from build123d import *

# Parameters (mm, degrees)
F0_R        = 5.8
F0_R_2      = 1.1
F1_DEPTH    = 2.5
F2_R        = 0.65
F3_DEPTH    = 25
F5_T2_ANGLE = 77.9776147156
F5_T4_ANGLE = 162.2494051266
F5_T6_ANGLE = 155.9758879551
F5_T8_ANGLE = 84.2484124222


# Not quite as in the source:
# - a fillet or chamfer that OpenCascade refuses, or shapes differently, is made with other operations: its cross-section is extruded or revolved along the edge and cut away or added


with BuildPart() as f1:
    # F0 (on Top) → F1 (new body)
    with BuildSketch(Plane.XY):
        Circle(F0_R)
        Circle(F0_R_2, mode=Mode.SUBTRACT)
    extrude(amount=F1_DEPTH)

    # F2 (on face) → F3 (cut)
    with BuildSketch(Plane.XY.offset(2.5)):
        with Locations((-4, 0)):
            Circle(F2_R)
        with Locations((2.125, 3.3888604279)):
            Circle(F2_R)
        with Locations((1.7421875, -3.6006642047)):
            Circle(F2_R)
    extrude(amount=-F3_DEPTH, mode=Mode.SUBTRACT)

    # F4: chamfer of 1.75 on 1 edges, made by hand

    # F4_s1 → F4_t2 (revolve, cut)
    with BuildSketch(Plane.XZ):
        Polygon((5.8, 0.75), (4.05, 2.5), (5.8, 2.5), align=None)
    revolve(axis=Axis((0, 0, 2.5), (0, 0, 1)), mode=Mode.SUBTRACT)

    # F5: fillet of radius 2 on 4 edges, made by hand

    # F5_s1 → F5_t2 (revolve, cut)
    with BuildSketch(Plane.XZ):
        with BuildLine():
            ThreePointArc((4.6357864376, 1.9142135624), (3.98693974, 2.347759065), (3.2215728753, 2.5))
            Line((3.2215728753, 2.5), (4.05, 2.5))
            Line((4.05, 2.5), (4.6357864376, 1.9142135624))
        make_face()
    revolve(axis=Axis((0, 0, 2.5), (0, 0, 1)), revolution_arc=F5_T2_ANGLE, mode=Mode.SUBTRACT)

    # F5_s3 → F5_t4 (revolve, cut)
    with BuildSketch(Plane(origin=(0, 0, 0), x_dir=(0, 0, 1), z_dir=(0.61332513, -0.7898305419, 0))):
        with BuildLine():
            ThreePointArc((1.9142135624, -4.6357864376), (2.347759065, -3.98693974), (2.5, -3.2215728753))
            Line((2.5, -3.2215728753), (2.5, -4.05))
            Line((2.5, -4.05), (1.9142135624, -4.6357864376))
        make_face()
    revolve(axis=Axis((0, 0, 2.5), (0, 0, 1)), revolution_arc=F5_T4_ANGLE, mode=Mode.SUBTRACT)

    # F5_s5 → F5_t6 (revolve, cut)
    with BuildSketch(Plane(origin=(0, 0, 0), x_dir=(0, 0, 1), z_dir=(0.3432973656, 0.9392267664, 0))):
        with BuildLine():
            ThreePointArc((1.9142135624, -4.6357864376), (2.347759065, -3.98693974), (2.5, -3.2215728753))
            Line((2.5, -3.2215728753), (2.5, -4.05))
            Line((2.5, -4.05), (1.9142135624, -4.6357864376))
        make_face()
    revolve(axis=Axis((0, 0, 2.5), (0, 0, 1)), revolution_arc=F5_T6_ANGLE, mode=Mode.SUBTRACT)

    # F5_s7 → F5_t8 (revolve, cut)
    with BuildSketch(Plane(origin=(0, 0, 0), x_dir=(0, 0, 1), z_dir=(-0.9949657418, -0.1002156306, 0))):
        with BuildLine():
            ThreePointArc((1.9142135624, -4.6357864376), (2.347759065, -3.98693974), (2.5, -3.2215728753))
            Line((2.5, -3.2215728753), (2.5, -4.05))
            Line((2.5, -4.05), (1.9142135624, -4.6357864376))
        make_face()
    revolve(axis=Axis((0, 0, 2.5), (0, 0, 1)), revolution_arc=F5_T8_ANGLE, mode=Mode.SUBTRACT)


solid = f1.part
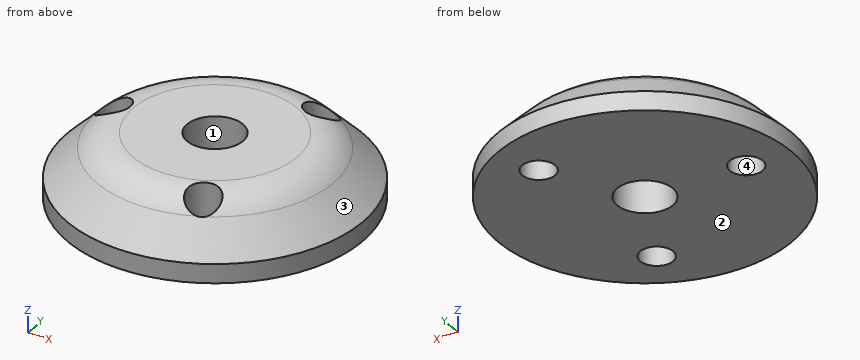
Check sheet for the modelled part. Datum: model origin and axes. Units: mm. Face numbers are marked on the shaded views. Give positions to 0.01 mm unless a question says otherwise; leave off trailing zeros. Order: outer loops, then holes, each group sorted by start corner. A loop starts at its lowest first (then second) coordinate and runs counter-clockwise, first axis right, second up. Notation, with made-up numbers: M -38.5,52.5 L -23.5,52.5 A21 cw -23.5,85.5 Z; hole C -2,42 d2. An arc over 180 degrees is marked long. Answer as CSV lines item,"result". Start each with the question number.
Item 1: Gauge pin test, flat ends, axial feed: P1, Ø1.5, axis at x = 1.5, z = 0.5, coming from the +Y side; P2, Ø1, axis at x = 1, z = 1, coming from the -Y side. Record the tip position at first contact, or that the pin passes through.
Item 2: Thickness scan on line 1 (Y direction, x = 0, z = 0.6); line 2 (Y direction, x = -4.25, z = 1.35); line 3 (Z direction, x = 4.25, y = 3.5). Record the ranges inside material, lowest first. Write a range as [from, to].
Item 3: Mould release check, pull along Y, two halves, no side actions. Record for the marked faces 1, 2, 3 and 4: +Y half, -Y half, draft (parallel to the pull), parting line (faces both ways), or undercut.
Item 4: Cross-section at B-B on y = 0. Enter the section's corners in (x, z), plus the area to 3 significant figures.
Item 5: Cross-section at C-C on z = 1.35. Enter the section's corners in (x, y) (3 decimals), plus the area to 3 significant figures.
Item 6: Cross-section at A-A on x = 0. Enter the section's corners in (y, z), plus the area to 3 significant figures.
Established:
1,P1,"stops at y = 5.75"
1,P2,"stops at y = -5.77"
2,line 1,"y = [-5.8, -1.1], [1.1, 5.8]"
2,line 2,"y = [-3, -0.6], [0.6, 3]"
2,line 3,"z = [0, 1.04]"
3,face 1,"undercut"
3,face 2,"draft"
3,face 3,"parting line"
3,face 4,"undercut"
4,outline,"M -5.8,0 L -4.65,0 L -4.65,1.9 L -5.8,0.75 Z; M -3.35,0 L -1.1,0 L -1.1,2.5 L -3.22,2.5 A2 ccw -3.35,2.5 Z; M 1.1,0 L 5.8,0 L 5.8,0.75 L 4.64,1.91 A2 ccw 3.22,2.5 L 1.1,2.5 Z"
4,area,"17.3 mm^2"
5,outline,"C 0,0 d10.4; hole C -4,0 d1.3; hole C 0,0 d2.2; hole C 1.742,-3.601 d1.3; hole C 2.125,3.389 d1.3"
5,area,"77.2 mm^2"
6,outline,"M -5.8,0 L -1.1,0 L -1.1,2.5 L -3.22,2.5 A2 ccw -4.64,1.91 L -5.8,0.75 Z; M 1.1,0 L 5.8,0 L 5.8,0.75 L 4.64,1.91 A2 ccw 3.22,2.5 L 1.1,2.5 Z"
6,area,"20.3 mm^2"
